Geometry check sheet. Reference: drawing and pictorial views, mm from the part's lowest x, y, z. Give positions to 0.01 mm unless a question says otherwise; leave off trailing zeros. Write each loop counter-clockwise with the first axis right and the second up, starting at its lowest first coordinate (ties: lowest second). Pieces come first, ordered by that corner, then holes. Notation, with made-up numbers: (37.25, 83) -> (60.25, 83) arc R26 cw to (60.25, 99) -> close; hole circle Ø7 at (-28.5, 43). An arc over 180 degrees is marked (long way). Use a Markdown table: item, result. Add a question column.
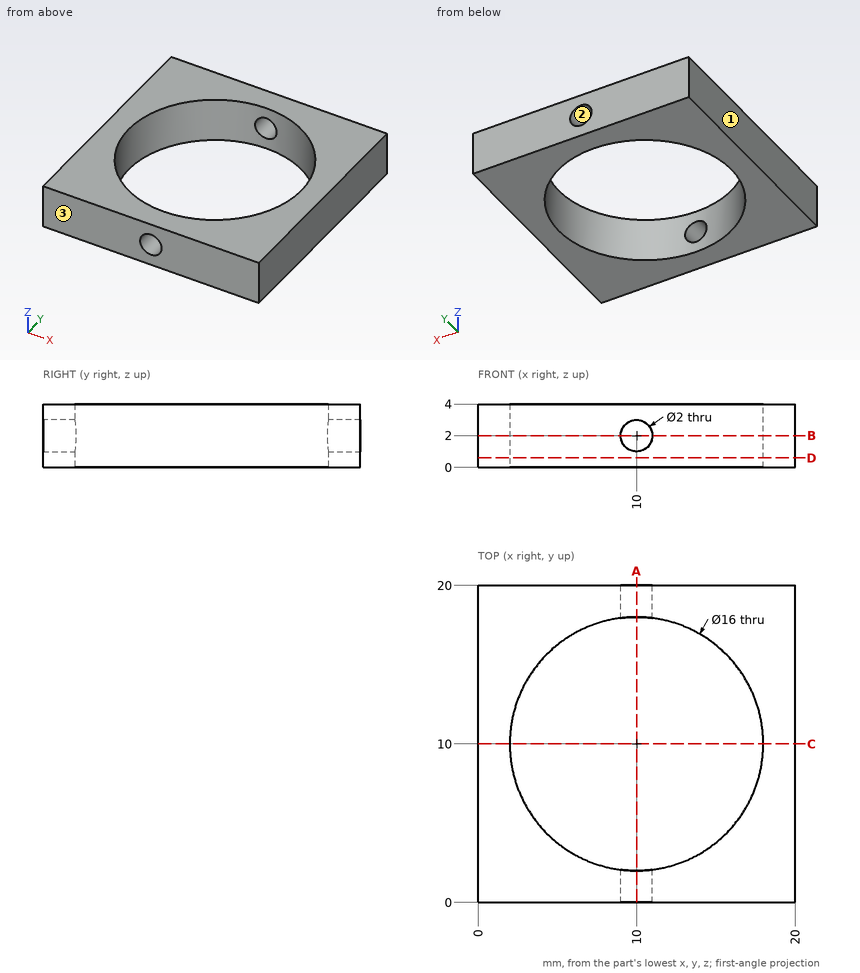
1) Sectioned sample at B-B, the plane z = 2. Enter the section's corners in (x, y), and give its area (3 significant figures).
2) Draft check along X on the marked faces 1, 2 and 3. Enter one of: +X half, -X half, draft (parallel to the pull), parting line (faces both ways), or undercut.
3) Material ranges on probe 1 along Z at (x, y) = (10, 0.8); probe 2 along Y at (x, z) = (9, 3.1); probe 3 along X at (y, z) = (1.4, 2), recorded low to high. Write a range as [from, to].
4) Sectioned sample at A-A, the plane x = 10. Enter the section's corners in (y, z).
5) Sectioned sample at D-D, the plane z = 0.6. Enter the section's corners in (x, y), and give its area (3 significant figures).
6) Sectioned sample at C-C, the plane y = 10. Enter the section's corners in (x, z), and give its area (3 significant figures).
Check values:
| question | item | result |
|---|---|---|
| 1 | outline | (0, 0) -> (9, 0) -> (9, 2.06) arc R8 cw to (9, 17.94) -> (9, 20) -> (0, 20) -> close; (11, 0) -> (20, 0) -> (20, 20) -> (11, 20) -> (11, 17.94) arc R8 cw to (11, 2.06) -> close |
| 1 | area | 191 mm² |
| 2 | face 1 | -X half |
| 2 | face 2 | undercut |
| 2 | face 3 | draft |
| 3 | probe 1 | [0, 1], [3, 4] |
| 3 | probe 2 | [0, 2.06], [17.94, 20] |
| 3 | probe 3 | [0, 9], [11, 20] |
| 4 | outline | (0, 0) -> (2, 0) -> (2, 1) -> (0, 1) -> close; (0, 3) -> (2, 3) -> (2, 4) -> (0, 4) -> close; (18, 0) -> (20, 0) -> (20, 1) -> (18, 1) -> close; (18, 3) -> (20, 3) -> (20, 4) -> (18, 4) -> close |
| 5 | outline | (0, 0) -> (20, 0) -> (20, 20) -> (0, 20) -> close; hole circle Ø16 at (10, 10) |
| 5 | area | 199 mm² |
| 6 | outline | (0, 0) -> (2, 0) -> (2, 4) -> (0, 4) -> close; (18, 0) -> (20, 0) -> (20, 4) -> (18, 4) -> close |
| 6 | area | 16.0 mm² |
